The figure shows three views and two pictorial views of one solid part (mm, origin at its lowest corner). Answer the questions. A direction names the side the tool comes from. Coordinates: 2 decimals unless noted, no trailing zeros. Loops run counter-clockwise (first coordinate to the right, second up) from the corner with the lowest first, then second, coordinate; pieces in that order, holes last. Notation, with made-up numbers: (-32.5, 34.25) -> (25.5, 34.25) arc R12 ccw to (25.5, 56.25) -> close; hole circle Ø1 at (86.25, 35). An arc over 180 degrees is marked (long way). Answer in a Markdown table with one row per item.
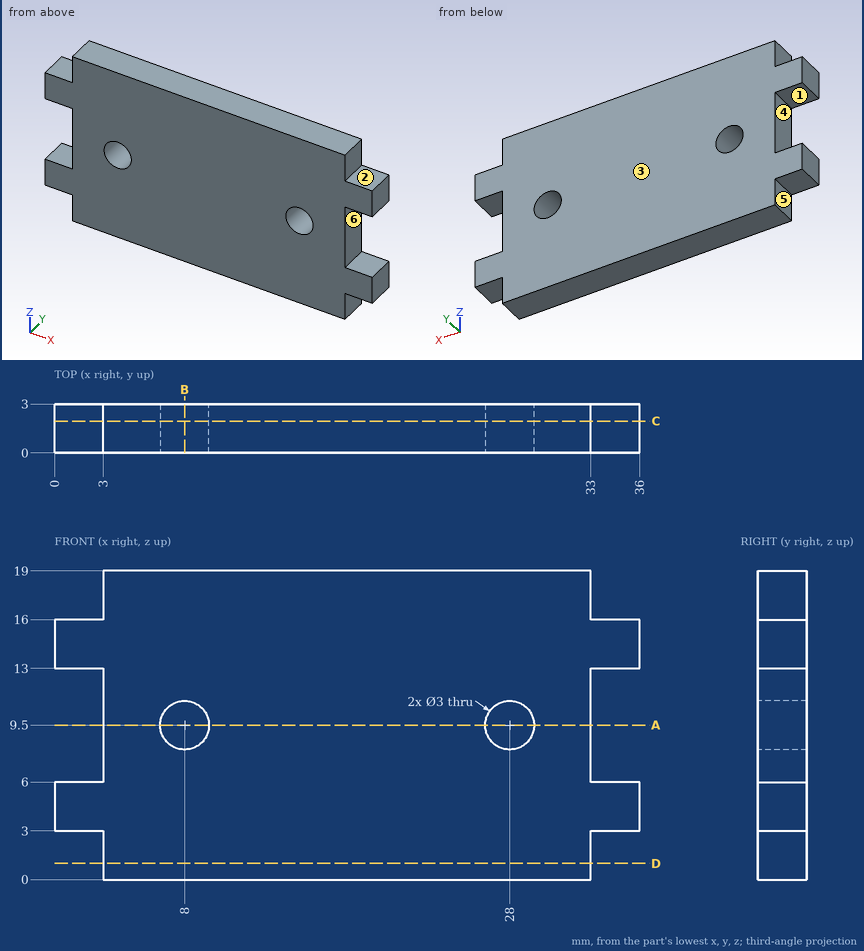
Item 1: Find the intervals of material crossed by probe 1 along X at (y, z) = (2, 9.5); probe 2 along Z at (x, y) = (28, 2.1); probe 3 along Z at (x, y) = (34, 2.6), in increasing order.
Findings below:
| item | result |
|---|---|
| probe 1 | x = 3 to 6.5, 9.5 to 26.5, 29.5 to 33 |
| probe 2 | z = 0 to 8, 11 to 19 |
| probe 3 | z = 3 to 6, 13 to 16 |
Item 2: A cutting plane is placed at D-D, the plane z = 1. Determine the outline of the cut face in (x, y).
Findings below:
| item | result |
|---|---|
| outline | (3, 0) -> (33, 0) -> (33, 3) -> (3, 3) -> close |
Item 3: Flat-ended cylindrical pins translate along their axes: pin 1 Ø0.9 at (x, y) = (34, 1) entering from +Z; pin 2 Ø2.5 at (x, z) = (28, 9.5) entering from -Y; pin 3 Ø1 at (x, z) = (18, 8) entering from -Y; pin 4 Ø0.9 at (x, y) = (34, 1) entering from -Z. Find the tip coordinate at first contact, or state that the pin passes through.
Findings below:
| item | result |
|---|---|
| pin 1 | stops at z = 16 |
| pin 2 | passes through |
| pin 3 | stops at y = 0 |
| pin 4 | stops at z = 3 |
Item 4: A cutting plane is placed at C-C, the plane y = 1.95. Determine the outline of the cut face in (x, z), plus the area to 3 significant figures.
Findings below:
| item | result |
|---|---|
| outline | (0, 3) -> (3, 3) -> (3, 0) -> (33, 0) -> (33, 3) -> (36, 3) -> (36, 6) -> (33, 6) -> (33, 13) -> (36, 13) -> (36, 16) -> (33, 16) -> (33, 19) -> (3, 19) -> (3, 16) -> (0, 16) -> (0, 13) -> (3, 13) -> (3, 6) -> (0, 6) -> close; hole circle Ø3 at (8, 9.5); hole circle Ø3 at (28, 9.5) |
| area | 592 mm2 |
Item 5: A cutting plane is placed at A-A, the plane z = 9.5. Determine the outline of the cut face in (x, y).
Findings below:
| item | result |
|---|---|
| outline | (3, 0) -> (6.5, 0) -> (6.5, 3) -> (3, 3) -> close; (9.5, 0) -> (26.5, 0) -> (26.5, 3) -> (9.5, 3) -> close; (29.5, 0) -> (33, 0) -> (33, 3) -> (29.5, 3) -> close |
Item 6: Determine the mould class of the marked faces 1, 2 and 3 for opening direction Z: +Z half, -Z half, draft (parallel to the pull), parting line (faces both ways), or undercut.
Findings below:
| item | result |
|---|---|
| face 1 | undercut |
| face 2 | +Z half |
| face 3 | draft |
Item 7: A tool of negligible diameter and unlimited length cuts with its end or side. For the marked faces 4, 5 and 6, from which of +Z, -Z, +X, -X, +Y, -Y can it reach the whole face along a straight path? Write none if from no direction.
Findings below:
| item | result |
|---|---|
| face 4 | -X, +Y, -Y |
| face 5 | -Z, -X, +Y, -Y |
| face 6 | +X, +Y, -Y |
Item 8: A cutting plane is placed at B-B, the plane x = 8. Determine the outline of the cut face in (y, z), plus the area to 3 significant figures.
Findings below:
| item | result |
|---|---|
| outline | (0, 0) -> (3, 0) -> (3, 8) -> (0, 8) -> close; (0, 11) -> (3, 11) -> (3, 19) -> (0, 19) -> close |
| area | 48.0 mm2 |
